Input: part model. Units: mm. Frame: model coordinates. Give positions to 0.01 mm unless a question says otherwise; leave off trailing zeros. Loops run counter-clockwise (first coordinate to the right, second up) from the corner with the lowest first, then second, coordinate; pieces in that order, holes last. Notation, with made-up numbers: M -20,73.5 L 17,73.5 A30 ccw 17,108.5 Z; hole C 59,83 d5. An arc over 180 degrees is marked long. Return JSON: item names as keys, results as strings. Group by question number.
```python
from build123d import *

# Parameters (mm, degrees)
BOSS_EXTRUDE1_DEPTH = 15


with BuildPart() as part:
    # Sketch1 → Boss-Extrude1 (new body)
    with BuildSketch(Plane.XY):
        with BuildLine():
            Line((0, 0), (100, 0))
            Line((100, 0), (100, 190))
            ThreePointArc((100, 190), (97.071067812, 197.071067812), (90, 200))
            Line((90, 200), (60, 200))
            Line((60, 200), (-1.149354388, 119.153849333))
            ThreePointArc((-1.149354388, 119.153849333), (39.497953664, 65.553662986), (-10, 20))
            Line((-10, 20), (-10, 10))
            Line((-10, 10), (0, 0))
        make_face()
    extrude(amount=BOSS_EXTRUDE1_DEPTH)


solid = part.part
```
Item 1: Section D-D, the plane y = 175. Return loops of the section in (x, z), then the cut area to 3 significant figures.
Item 2: Section C-C, the plane x = 27. Return loops of the section in (y, z), then the cut area to 3 significant figures.
Item 3: Material intervals for line 1 (Y direction, x = 27.5, z = 8.5); line 2 (Y direction, x = 10, z = 4); line 3 (X direction, y = 148.5, z = 12.25), sorted ascending. Write a range as from..to.
Item 4: Section B-B, the plane x = 5. Return loops of the section in (y, z).
Item 5: Section A-A, the plane z = 10.5. Return loops of the section in (x, y), then the cut area to 3 significant figures.
Item 6: First-contact query: pin 1 Ø2 at (y, z) = (169.5, 7.5) entering from -X; pin 2 Ø2 at (x, z) = (14.5, 6) entering from +Y; pin 3 Ø6 at (y, z) = (46.5, 12.5) entering from -X. Flat tips, straight axial feed; report the tip coordinate or a pass-through.
Answer below:
{
 "1": {"outline": "M 41.09,0 L 100,0 L 100,15 L 41.09,15 Z", "area": "884 mm^2"},
 "2": {"outline": "M 0,0 L 36.71,0 L 36.71,15 L 0,15 Z; M 103.29,0 L 156.37,0 L 156.37,15 L 103.29,15 Z", "area": "1,350 mm^2"},
 "3": {"line 1": "0..37.28, 102.72..157.03", "line 2": "0..24.31, 115.69..133.89", "line 3": "21.05..100"},
 "4": {"outline": "M 0,0 L 22.4,0 L 22.4,15 L 0,15 Z; M 117.6,0 L 127.28,0 L 127.28,15 L 117.6,15 Z"},
 "5": {"outline": "M -10,10 L 0,0 L 100,0 L 100,190 A10 ccw 90,200 L 60,200 L -1.15,119.15 A50 cw -10,20 Z", "area": "14,800 mm^2"},
 "6": {"pin 1": "x = 36.17", "pin 2": "y = 141.17", "pin 3": "x = 32.1"}
}
